Read the model definition and answer for the solid it produces. Units are mm, in the model's axes. A direction names the side the tool comes from. Coordinates: 2 decimals unless noted, no trailing zeros. Write each loop counter-clockwise with the first axis right and the second up, starting at its lowest first coordinate (ties: lowest second). Pieces come first, ordered by that corner, then holes.
(1) Section B-B on y = 0.4 is taken. Write down the section's boundary in (x, z), then the cut area to 3 significant figures.
(2) Section D-D on x = 4 is taken. Write down the section's boundary in (y, z), then the cut area to 3 significant figures.
(3) Given pin 1 (3 mm diameter, centred on x = -12, y = -0.5, fed in from -Z), flat-ended and moving along its own axis, determine where the tip first touches the part or whether it passes through.
(4) Which of the six approach directions +Z, -Z, +X, -X, +Y, -Y give full straight-line access (tool end or side, diameter ignored) to faces 5 (the flat face through (0, 0, 0)), 6 (the flat face through (14.9, 0, -6.6)), 7 (the cylindrical face through (-14.25, -0.04, -5.5))?
(5) Find the intervals of material crossed by probe 1 along X at (y, z) = (2.1, -4.5); probe 2 along Z at (x, y) = (8.5, 2.45); probe 3 along Z at (x, y) = (1, -0.55), in increasing order.
(6) Section A-A on z = -4 is taken. Write down the section's boundary in (x, y), then the cut area to 3 significant figures.
(7) The mould has two halves that part along Z. Classify faces 1 (the cylindrical face through (14.25, -0.04, -5.5)), 2 (the flat face through (5, 0, -4)), 3 (the flat face through (0, 0, -5)), 4 (the flat face through (-15.5, 0, -4)): +Z half, -Z half, draft (parallel to the pull), parting line (faces both ways), or undercut.
(8) Section C-C on x = -13 is taken. Write down the section's boundary in (y, z).
from build123d import *

# Parameters (mm, degrees)
F0_W     = 10
F0_H     = 2
F1_DEPTH = 3
F2_R     = 2
F3_R     = 0.5
F4_R     = 0.5


with BuildPart() as f1:
    # F0 (on Front) → F1 (new body, symmetric)
    with BuildSketch(Plane.XZ):
        Polygon((18.5, 0), (-18.5, 0), (-18.5, -7.2), (-15.5, -7.2), (-13.5, -5.2), (-15.5, -5.2), (-15.5, -3), (-5, -3), (5, -3), (15.5, -3), (15.5, -5.2), (13.5, -5.2), (15.5, -7.2), (18.5, -7.2), align=None)
        with Locations((0, -4)):
            Rectangle(F0_W, F0_H)
    extrude(amount=F1_DEPTH, both=True)

    # F2
    f2_edges = [f1.edges().sort_by_distance(p)[0] for p in [
        (18.5, 0, 0),
        (-18.5, 0, 0),
    ]]
    fillet(f2_edges, radius=F2_R)

    # F3
    f3_edges = [f1.edges().sort_by_distance(p)[0] for p in [
        (15.5, 0, -3),
        (-15.5, 0, -3),
    ]]
    fillet(f3_edges, radius=F3_R)

    # F4
    f4_edges = [f1.edges().sort_by_distance(p)[0] for p in [
        (13.5, 0, -5.2),
        (-13.5, 0, -5.2),
    ]]
    fillet(f4_edges, radius=F4_R)


solid = f1.part
Response:
1. outline: (-18.5, -7.2) - (-15.5, -7.2) - (-14.35, -6.05) arc R0.5 ccw to (-14.71, -5.2) - (-15.5, -5.2) - (-15.5, -3.5) arc R0.5 cw to (-15, -3) - (-5, -3) - (-5, -5) - (5, -5) - (5, -3) - (15, -3) arc R0.5 cw to (15.5, -3.5) - (15.5, -5.2) - (14.71, -5.2) arc R0.5 ccw to (14.35, -6.05) - (15.5, -7.2) - (18.5, -7.2) - (18.5, -2) arc R2 ccw to (16.5, 0) - (-16.5, 0) arc R2 ccw to (-18.5, -2) - close
1. area: 158 mm2
2. outline: (-3, -5) - (3, -5) - (3, 0) - (-3, 0) - close
2. area: 30.0 mm2
3. pin 1: stops at z = -3
4. face 5: +Z, +X, -X, +Y, -Y
4. face 6: -Z, +Y, -Y
4. face 7: +Y, -Y
5. probe 1: x = -18.5 to -15.5, -5 to 5, 15.5 to 18.5
5. probe 2: z = -3 to 0
5. probe 3: z = -5 to 0
6. outline: (-18.5, -3) - (-15.5, -3) - (-15.5, 3) - (-18.5, 3) - close; (-5, -3) - (5, -3) - (5, 3) - (-5, 3) - close; (15.5, -3) - (18.5, -3) - (18.5, 3) - (15.5, 3) - close
6. area: 96.0 mm2
7. face 1: undercut
7. face 2: draft
7. face 3: -Z half
7. face 4: undercut
8. outline: (-3, -3) - (3, -3) - (3, 0) - (-3, 0) - close
